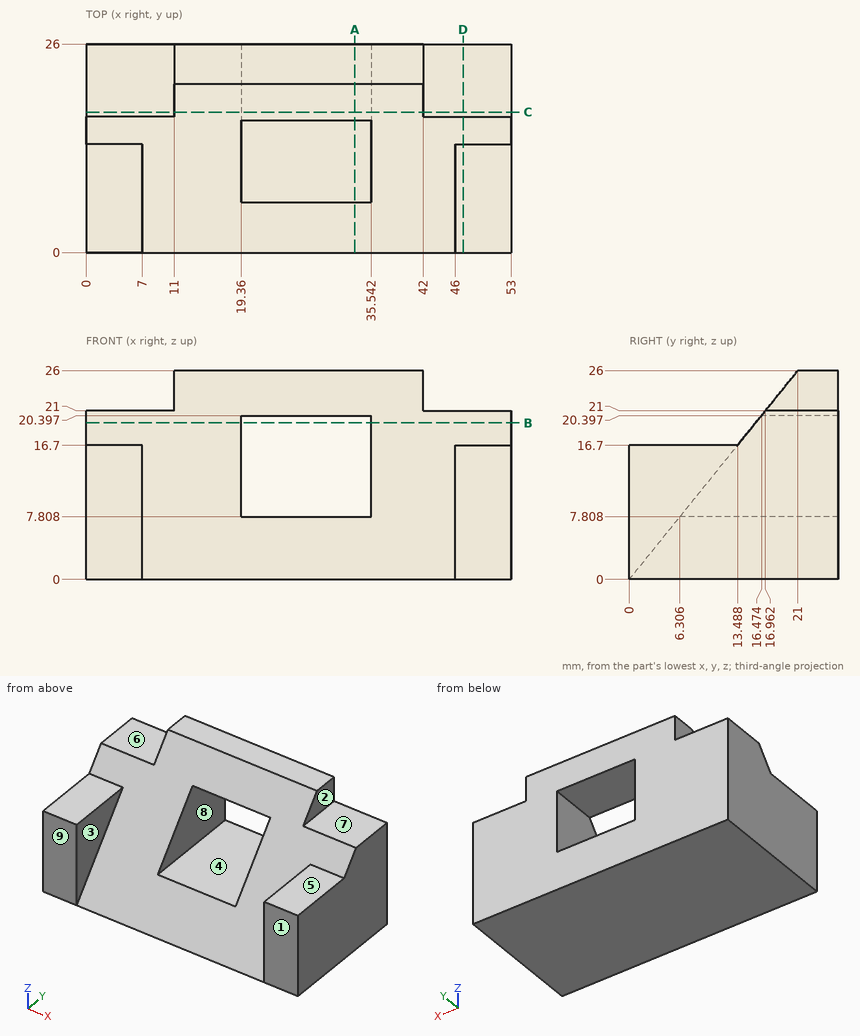
Design review of the part shown in the three views and the two pictorial views. Dimensions are in mm from the part's minimum x, y and z. A direction names the side the tool comes from. Round coordinates to 2 decimals unless told otherwise and drop trailing zeros. Write each loop counter-clockwise with the first axis right and the second up, starting at its lowest first coordinate (ties: lowest second). Pieces come first, ordered by that corner, then holes.
1) Take a section at B-B on z = 19.5. Give the boundary of the cut face in (x, y).
Answer below:
outline: (0, 15.75) - (19.36, 15.75) - (19.36, 26) - (0, 26) - close; (35.54, 15.75) - (53, 15.75) - (53, 26) - (35.54, 26) - close
2) For line 1 along X through (y, z) = (20.5, 11.5); line 2 along Z through (x, y) = (24, 24.5); line 3 along Z through (x, y) = (21.5, 18.75) (1 decimal), list the stretches that pass through material, from the lowest coordinate up.
Answer below:
line 1: x = 0 to 19.36, 35.54 to 53
line 2: z = 0 to 7.81, 20.4 to 26
line 3: z = 0 to 7.8, 20.4 to 23.2
3) Take a section at D-D on x = 47. Give the boundary of the cut face in (y, z).
Answer below:
outline: (0, 0) - (26, 0) - (26, 21) - (16.96, 21) - (13.49, 16.7) - (0, 16.7) - close
4) Insertion check: pin 1 Ø4 at (x, z) = (39.5, 12.5) entering from -Y; pin 2 Ø2.5 at (x, y) = (5, 22) entering from +Z; pin 3 Ø3.5 at (x, y) = (48.5, 8.5) entering from +Z. Each pin has a flat end and moves straight along its axis. Give the tip position at first contact, or say it passes through.
Answer below:
pin 1: stops at y = 8.48
pin 2: stops at z = 21
pin 3: stops at z = 16.7
5) Take a section at A-A on x = 33.5. Give the boundary of the cut face in (y, z) (1 decimal).
Answer below:
outline: (0, 0) - (26, 0) - (26, 7.8) - (6.3, 7.8) - close; (16.5, 20.4) - (26, 20.4) - (26, 26) - (21, 26) - close
6) Machinability: for the marked faces 5, 6, 7, 8 and 9, which of the approach directions +Z, -Z, +X, -X, +Y, -Y give a long, thin tool a straight path to every point of the face, cutting with its end or side? Answer none if there is none.
Answer below:
face 5: +Z, +X, -X, -Y
face 6: +Z, -X, +Y, -Y
face 7: +Z, +X, +Y, -Y
face 8: +Y, -Y
face 9: +Z, -Z, +X, -X, -Y
7) Mouldability with a two-part tool opening along X and no side actions: class the marked faces 1, 2, 3 and 4 as +X half, -X half, draft (parallel to the pull), parting line (faces both ways), or undercut.
Answer below:
face 1: draft
face 2: +X half
face 3: undercut
face 4: undercut
8) Take a section at C-C on y = 17.5. Give the boundary of the cut face in (x, z).
Answer below:
outline: (0, 0) - (53, 0) - (53, 21) - (42, 21) - (42, 21.67) - (11, 21.67) - (11, 21) - (0, 21) - close; hole (19.36, 7.81) - (35.54, 7.81) - (35.54, 20.4) - (19.36, 20.4) - close
